Input: part model. Units: mm. Frame: model coordinates. Coordinates: 2 decimals unless noted, no trailing zeros. Write each loop counter-clockwise with the first axis right and the second up, starting at its lowest first coordinate (ties: lowest second). Pieces come first, ordered by that corner, then holes.
1) Pin query (flat end, axial travel): pin 1 Ø1 at (x, y) = (68, -4.5) entering from +Z. Return the tip coordinate at first contact, or that it passes through.
2) Section query C-C (y = -0.95). Output: boundary loops of the cut face in (x, z).
3) Section query B-B (x = 120). Output: boundary loops of the cut face in (y, z), then the cut area to 3 significant figures.
4) Section query A-A (x = 10). Output: boundary loops of the cut face in (y, z), then the cut area to 4 significant figures.
5) Line query: L1, parallel to X at y = -2.2, z = 10; L2, parallel to Z at x = 8, y = -2.05; L3, parallel to X at y = -4.25, z = 19. Output: solid intervals per line, ascending.
6) Section query D-D (x = 96.5). Output: boundary loops of the cut face in (y, z).
from build123d import *

# Parameters (mm, degrees)
F0_R     = 3
F1_DEPTH = 5


with BuildPart() as f1:
    # F0 (on Front) → F1 (new body)
    with BuildSketch(Plane.XZ):
        with BuildLine():
            Line((0, 50.189292), (0, 0))
            Line((0, 0), (130, 0.007858))
            Line((130, 0.007858), (130, 29.081571))
            Line((130, 29.081571), (108.241631, 16.878763))
            ThreePointArc((108.241631, 16.878763), (107.581922, 16.487004), (106.903636, 16.128371))
            ThreePointArc((106.903636, 16.128371), (97.760054, 14.668749), (89.415819, 18.682392))
            Line((89.415819, 18.682392), (76.946103, 37.473632))
            Line((76.946103, 37.473632), (69.468242, 24.439426))
            ThreePointArc((69.468242, 24.439426), (68.444533, 22.28673), (67.102852, 20.316458))
            ThreePointArc((67.102852, 20.316458), (57.214619, 14.659027), (46.130044, 17.288828))
            Line((46.130044, 17.288828), (3.445965, 47.074116))
            ThreePointArc((3.445965, 47.074116), (1.605618, 48.501877), (0, 50.189292))
        make_face()
        with Locations((10, 10.000604)):
            Circle(F0_R, mode=Mode.SUBTRACT)
        with Locations((70, 8.004231)):
            Circle(F0_R, mode=Mode.SUBTRACT)
        with Locations((120, 10.007253)):
            Circle(F0_R, mode=Mode.SUBTRACT)
        with Locations((78, 20.004715)):
            Circle(F0_R, mode=Mode.SUBTRACT)
        with Locations((10, 32.000605)):
            Circle(F0_R, mode=Mode.SUBTRACT)
    extrude(amount=F1_DEPTH)


solid = f1.part
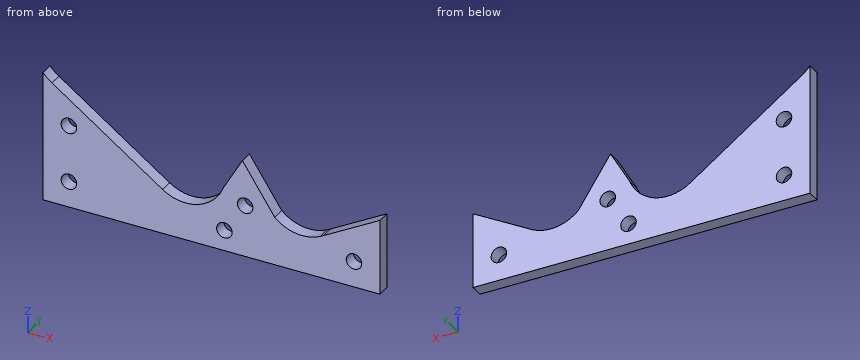
Answer:
1. pin 1: stops at z = 22.38
2. outline: (0, 0) - (130, 0.01) - (130, 29.08) - (108.24, 16.88) arc R15.5 cw to (106.9, 16.13) arc R15.5 cw to (89.42, 18.68) - (76.95, 37.47) - (69.47, 24.44) arc R15.5 cw to (67.1, 20.32) arc R15.5 cw to (46.13, 17.29) - (3.45, 47.07) arc R15.5 cw to (0, 50.19) - close; hole circle Ø6 at (10, 10); hole circle Ø6 at (10, 32); hole circle Ø6 at (70, 8); hole circle Ø6 at (78, 20); hole circle Ø6 at (120, 10.01)
3. outline: (-5, 0.01) - (0, 0.01) - (0, 7.01) - (-5, 7.01) - close; (-5, 13.01) - (0, 13.01) - (0, 23.47) - (-5, 23.47) - close
3. area: 87.3 mm2
4. outline: (-5, 0) - (0, 0) - (0, 7) - (-5, 7) - close; (-5, 13) - (0, 13) - (0, 29) - (-5, 29) - close; (-5, 35) - (0, 35) - (0, 42.5) - (-5, 42.5) - close
4. area: 152.5 mm2
5. L1: x = 0 to 7, 13 to 67.76, 72.24 to 117, 123 to 130
5. L2: z = 0 to 7.76, 12.24 to 29.76, 34.24 to 43.9
5. L3: x = 0 to 43.68, 65.92 to 75.17, 80.83 to 89.21, 112.02 to 130
6. outline: (-5, 0.01) - (0, 0.01) - (0, 14.91) - (-5, 14.91) - close
